Part print with two shaded views. Sizes in mm from the minimum x, y, z corner. A direction names the side the tool comes from. Round coordinates to 2 decimals unless told otherwise and drop trailing zeros. Order: outer loops, then holes, each group sorted by start corner. A loop starts at its lowest first (then second) coordinate and runs counter-clockwise, first axis right, second up. Notation, with made-up numbers: M -11.5,59.25 L 9.5,59.25 A22 ccw 9.5,78.25 Z; hole C 87,55.5 d5. An arc over 180 degrees is marked long. Put each result on its own line as item: value.
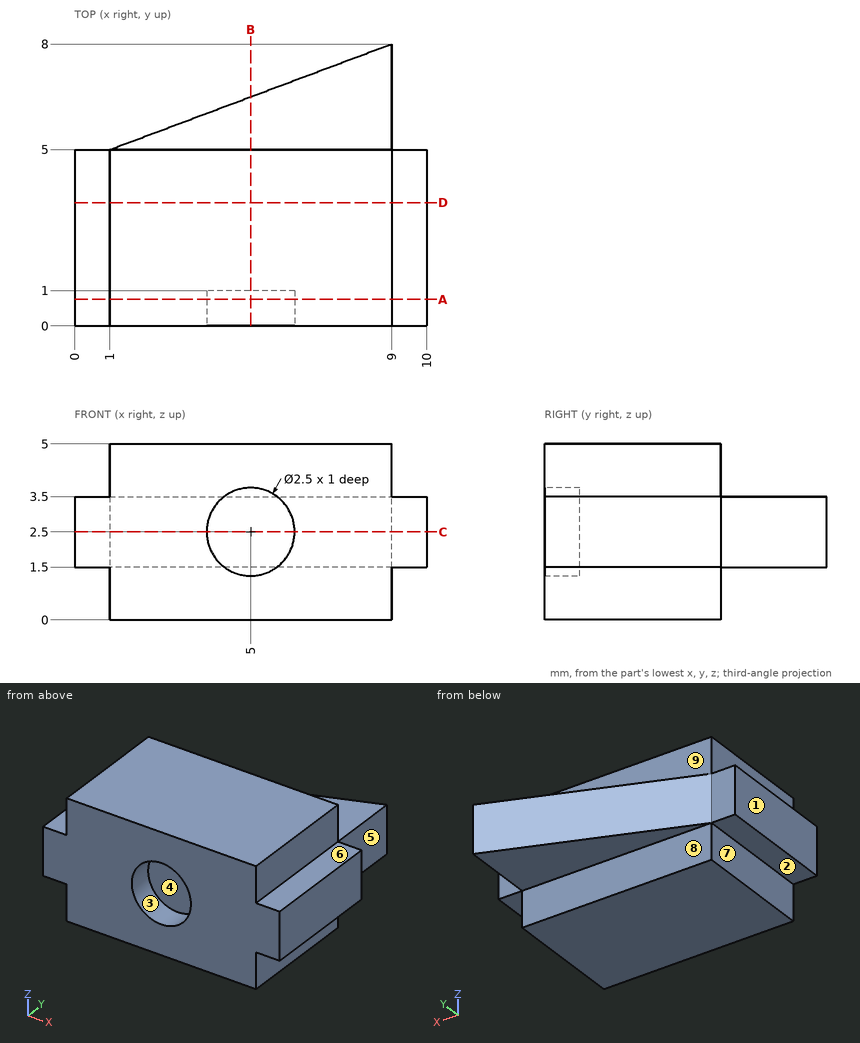
Item 1: Band-saw the part on D-D on y = 3.5. Give the cut face in (x, z).
Answers below:
outline: M 0,1.5 L 1,1.5 L 1,0 L 9,0 L 9,1.5 L 10,1.5 L 10,3.5 L 9,3.5 L 9,5 L 1,5 L 1,3.5 L 0,3.5 Z
Item 2: Pin check, flat tips, straight feed: P1, Ø1.2, axis at y = 2.5, z = 1, coming from the -X side; P2, Ø0.8, axis at y = 2, z = 0.5, coming from the +X side; P3, Ø0.5, axis at x = 9.5, y = 2, coming from the -Z side; P4, Ø0.5, axis at x = 0.5, y = 3, coming from the +Z side. Stop position of each tip, or through.
Answers below:
P1: x = 0
P2: x = 9
P3: z = 1.5
P4: z = 3.5
Item 3: Tool access for the marked faces 5, 6, 7, 8 and 9: list every direction of +Z, -Z, +X, -X, +Y, -Y with a clear straight run to the whole face (end or side of a thin tool).
Answers below:
face 5: +Z, -Z, +X, +Y
face 6: +Z, +X, +Y, -Y
face 7: -Z, -X, +Y, -Y
face 8: -Z, +X, -X, +Y
face 9: +Z, +X, -X, +Y
Item 4: Probe line 1 along X through (y, z) = (0.65, 2.5); line 2 along X through (y, z) = (3.5, 0.4); line 3 along Y through (x, z) = (8.25, 1.15). List the from-to ranges inside material, lowest first. Write a range as [from, to].
Answers below:
line 1: [0, 3.75], [6.25, 10]
line 2: [1, 9]
line 3: [0, 5]
Item 5: Mould opens along X. For the marked faces 1, 2, 3 and 4 say: pulls with the +X half, pulls with the -X half, needs draft (parallel to the pull), parting line crosses it, or undercut.
Answers below:
face 1: pulls with the -X half
face 2: needs draft
face 3: undercut
face 4: undercut
Item 6: Band-saw the part on A-A on y = 0.75. Give the cut face in (x, z).
Answers below:
outline: M 0,1.5 L 1,1.5 L 1,0 L 9,0 L 9,1.5 L 10,1.5 L 10,3.5 L 9,3.5 L 9,5 L 1,5 L 1,3.5 L 0,3.5 Z; hole C 5,2.5 d2.5
Item 7: Band-saw the part on B-B on x = 5. Give the cut face in (y, z), and give its area (3 significant figures).
Answers below:
outline: M 0,0 L 5,0 L 5,1.5 L 6.5,1.5 L 6.5,3.5 L 5,3.5 L 5,5 L 0,5 L 0,3.75 L 1,3.75 L 1,1.25 L 0,1.25 Z
area: 25.5 mm²
Item 8: Band-saw the part on C-C on z = 2.5. Give the cut face in (x, y).
Answers below:
outline: M 0,0 L 3.75,0 L 3.75,1 L 6.25,1 L 6.25,0 L 10,0 L 10,5 L 9,5 L 9,8 L 1,5 L 0,5 Z
